For this review, take the finished solid that the model builds, in its own axes (mm). A direction names the side the tool comes from. Round coordinates to 2 decimals unless told otherwise and drop trailing zeros. Order: outer loops, then holes, each group sorted by start corner. A loop starts at its lowest first (then second) coordinate and runs counter-clockwise, first axis right, second up. Notation, with made-up numbers: M 7.25,60 L 64.25,60 A19 cw 64.25,82 Z; hole C 6.5,64.5 d3. An arc over 180 degrees is marked long. Answer as a JSON object with one key per item and string values.
from build123d import *

# Parameters (mm, degrees)
SKETCH_R      = 12.3
EXTRUDE_DEPTH = 5
BOX001_W      = 82
BOX001_H      = 58
BOX001_DEPTH  = 44.4
BOX_W         = 74.7
BOX_H         = 38.74
BOX_DEPTH     = 44.4


with BuildPart() as extrude_body:
    # Sketch (on Face6 of Box001) → Extrude (new body)
    with BuildSketch(Plane(origin=(-82, -9.63, 44.4), x_dir=(1, 0, 0), z_dir=(0, 0, 1))):
        with Locations((23.3, 30)):
            Circle(SKETCH_R)
    extrude(amount=EXTRUDE_DEPTH)


with BuildPart() as cube001:
    # Box001 → Box001 (new body)
    with BuildSketch(Plane(origin=(-82, -9.63, 0), x_dir=(1, 0, 0), z_dir=(0, 0, 1))):
        with Locations((41, 29)):
            Rectangle(BOX001_W, BOX001_H)
    extrude(amount=BOX001_DEPTH)


with BuildPart() as fusion002:
    # Box → Box (new body)
    with BuildSketch(Plane.XY):
        with Locations((37.35, 19.37)):
            Rectangle(BOX_W, BOX_H)
    extrude(amount=BOX_DEPTH)

    # Fusion: union Cube001
    add(cube001.part)

    # Fusion002: union Extrude body
    add(extrude_body.part)


solid = fusion002.part
1) Add section C-C on y = 42. State the section outline as (x, z) points.
Geometry check:
{"outline": "M -82,0 L 0,0 L 0,44.4 L -82,44.4 Z"}
2) Insertion check: P1, Ø4, axis at x = 57, z = 33, coming from the +Y side; P2, Ø17.5, axis at x = 7.5, y = 9, coming from the +Z side. Each pin has a flat end and moves straight along its axis. Give the tip position at first contact, or say it passes through.
Geometry check:
{"P1": "stops at y = 38.74", "P2": "stops at z = 44.4"}
3) Add section A-A on y = 20.37. State the section outline as (x, z) points, and give its area (3 significant figures).
Geometry check:
{"outline": "M -82,0 L 74.7,0 L 74.7,44.4 L -46.4,44.4 L -46.4,49.4 L -71,49.4 L -71,44.4 L -82,44.4 Z", "area": "7,080 mm²"}
4) Machinability: for faces 1 (the flat face through (0, 43, 22)), 2 (the cylindrical face through (-70.99, 20.91, 46.86)), 3 (the flat face through (0, -5, 22)), which of the approach directions +Z, -Z, +X, -X, +Y, -Y give a long, thin tool a straight path to every point of the face, cutting with its end or side? Answer none if there is none.
Geometry check:
{"face 1": "+Z, -Z, +X, +Y", "face 2": "+Z", "face 3": "+Z, -Z, +X, -Y"}
5) Add section D-D on x = 61. State the section outline as (y, z) points, and give its area (3 significant figures).
Geometry check:
{"outline": "M 0,0 L 38.74,0 L 38.74,44.4 L 0,44.4 Z", "area": "1,720 mm²"}
6) Add section B-B on x = -58.7. State the section outline as (y, z) points, and give its area (3 significant figures).
Geometry check:
{"outline": "M -9.63,0 L 48.37,0 L 48.37,44.4 L 32.67,44.4 L 32.67,49.4 L 8.07,49.4 L 8.07,44.4 L -9.63,44.4 Z", "area": "2,700 mm²"}
7) For L1, parallel to X at y = 39, z = 24.5; L2, parallel to X at y = 19.5, z = 46; L3, parallel to Z at x = -34.5, y = 35, list the stretches that pass through material, from the lowest coordinate up.
Geometry check:
{"L1": "x = -82 to 0", "L2": "x = -70.97 to -46.43", "L3": "z = 0 to 44.4"}
